```python
from build123d import *

# Parameters (mm, degrees)
SKETCH_1_R               = 9.5
EXTRUDE_2_DEPTH          = 10
CHAMFER_1_SIZE           = 0.5
CUT_EXTRUDE_1_DEPTH      = 10
SKETCH_3_R               = 2
CUT_EXTRUDE_2_DEPTH      = 10
CHAMFER_2_SIZE           = 0.5
SKETCH_5_R               = 2
CUT_EXTRUDE_3_DEPTH      = 10
CHAMFER_3_SIZE           = 0.5
SKETCH_9_R               = 2
EXTRUDE_3_DEPTH          = 10
SKETCH_10_R              = 2
CUT_EXTRUDE_6_DEPTH      = 10
PATTERN_CIRCULAR_2_COUNT = 4
SKETCH_11_R              = 1.5
CUT_EXTRUDE_7_DEPTH      = 251.99800796


with BuildPart() as part:
    # Sketch 1 → Extrude 2 (new body)
    with BuildSketch(Plane.XY):
        with BuildLine():
            Line((20.821645942, -9.5), (202.986114682, -9.5))
            ThreePointArc((202.986114682, -9.5), (210.231803055, -10.858648118), (216.493057341, -14.75))
            ThreePointArc((216.493057341, -14.75), (250, 0), (216.493057341, 14.75))
            ThreePointArc((216.493057341, 14.75), (210.231803055, 10.858648118), (202.986114682, 9.5))
            Line((202.986114682, 9.5), (21.63860854, 9.5))
            Line((21.63860854, 9.5), (16.904141504, 9.5))
            ThreePointArc((16.904141504, 9.5), (11.75918395, 10.173090993), (6.960528855, 12.147058824))
            ThreePointArc((6.960528855, 12.147058824), (3.490452231, 13.557903349), (-0.229510749, 13.998118617))
            ThreePointArc((-0.229510749, 13.998118617), (-13.878745314, -1.838594167), (3.423256182, -13.575025492))
            ThreePointArc((3.423256182, -13.575025492), (5.240755683, -12.982083033), (6.960528855, -12.147058824))
            ThreePointArc((6.960528855, -12.147058824), (11.75918395, -10.173090993), (16.904141504, -9.5))
            Line((16.904141504, -9.5), (20.821645942, -9.5))
        make_face()
        Circle(SKETCH_1_R, mode=Mode.SUBTRACT)
        with Locations((230, 0)):
            Circle(SKETCH_1_R, mode=Mode.SUBTRACT)
    extrude(amount=EXTRUDE_2_DEPTH)

    # Chamfer 1
    chamfer_1_edges = [part.edges().sort_by_distance(p)[0] for p in [
        (-9.5, 0, 0),
        (-9.5, 0, 10),
    ]]
    chamfer(chamfer_1_edges, length=CHAMFER_1_SIZE)

    # Sketch 2 → Cut-Extrude 1 (cut)
    with BuildSketch(Plane.XY.offset(10)):
        with BuildLine():
            Line((92.5, -6), (137.5, -6))
            ThreePointArc((137.5, -6), (143.5, 0), (137.5, 6))
            Line((137.5, 6), (92.5, 6))
            ThreePointArc((92.5, 6), (86.5, 0), (92.5, -6))
        make_face()
        with BuildLine():
            Line((157.5, -6), (202.5, -6))
            ThreePointArc((202.5, -6), (208.5, 0), (202.5, 6))
            Line((202.5, 6), (157.5, 6))
            ThreePointArc((157.5, 6), (151.5, 0), (157.5, -6))
        make_face()
        with BuildLine():
            Line((35, -6), (72.5, -6))
            ThreePointArc((72.5, -6), (78.5, 0), (72.5, 6))
            Line((72.5, 6), (35, 6))
            ThreePointArc((35, 6), (29, 0), (35, -6))
        make_face()
    extrude(amount=-CUT_EXTRUDE_1_DEPTH, mode=Mode.SUBTRACT)

    # Sketch 3 → Cut-Extrude 2 (cut)
    with BuildSketch(Plane.XY.offset(10)):
        with Locations((245, 0)):
            Circle(SKETCH_3_R)
        with Locations((237.5, 12.990381057)):
            Circle(SKETCH_3_R)
        with Locations((222.5, 12.990381057)):
            Circle(SKETCH_3_R)
    extrude(amount=-CUT_EXTRUDE_2_DEPTH, mode=Mode.SUBTRACT)

    # Chamfer 2
    chamfer_2_edges = [part.edges().sort_by_distance(p)[0] for p in [
        (220.5, 0, 10),
    ]]
    chamfer(chamfer_2_edges, length=CHAMFER_2_SIZE)

    # Sketch 5 → Cut-Extrude 3 (cut)
    with BuildSketch(Plane.XY.offset(10)):
        with Locations((215, 0)):
            Circle(SKETCH_5_R)
        with Locations((222.5, -12.990381057)):
            Circle(SKETCH_5_R)
        with Locations((237.5, -12.990381057)):
            Circle(SKETCH_5_R)
    extrude(amount=-CUT_EXTRUDE_3_DEPTH, mode=Mode.SUBTRACT)

    # Chamfer 3
    chamfer_3_edges = [part.edges().sort_by_distance(p)[0] for p in [
        (220.5, 0, 0),
    ]]
    chamfer(chamfer_3_edges, length=CHAMFER_3_SIZE)

    # Sketch 9 → Extrude 3 (add)
    with BuildSketch(Plane.XY.offset(10)):
        with Locations((215, 0)):
            Circle(SKETCH_9_R)
        with Locations((222.5, 12.990381057)):
            Circle(SKETCH_9_R)
        with Locations((237.5, 12.990381057)):
            Circle(SKETCH_9_R)
        with Locations((245, 0)):
            Circle(SKETCH_9_R)
        with Locations((237.5, -12.990381057)):
            Circle(SKETCH_9_R)
        with Locations((222.5, -12.990381057)):
            Circle(SKETCH_9_R)
    extrude(amount=-EXTRUDE_3_DEPTH)

    # Sketch 10 → Cut-Extrude 6 (cut)
    with BuildSketch(Plane.XY.offset(10)):
        with Locations((214.5, 0)):
            Circle(SKETCH_10_R)
    cut_extrude_6 = extrude(amount=-CUT_EXTRUDE_6_DEPTH, mode=Mode.SUBTRACT)

    # Pattern Circular 2: Cut-Extrude 6 ×4 about axis
    pattern_circular_2_axis = Axis((230, 0, 0), (0, 0, 1))
    for i in range(1, PATTERN_CIRCULAR_2_COUNT):
        add(cut_extrude_6.rotate(pattern_circular_2_axis, i * 360 / PATTERN_CIRCULAR_2_COUNT), mode=Mode.SUBTRACT)

    # Sketch 11 → Cut-Extrude 7 (cut, through all)
    with BuildSketch(Plane.XY.offset(10)):
        with Locations((17, 4)):
            Circle(SKETCH_11_R)
        with Locations((17, -4)):
            Circle(SKETCH_11_R)
    extrude(amount=-CUT_EXTRUDE_7_DEPTH, mode=Mode.SUBTRACT)


solid = part.part
```
CAD build for the part. Positions are in the model's coordinates, mm. A direction names the side the tool comes from. Give positions to 0.01 mm unless a question says otherwise; leave off trailing zeros. Write each loop counter-clockwise with the first axis right and the second up, starting at its lowest first coordinate (ties: lowest second). Pieces come first, ordered by that corner, then holes. Notation, with made-up numbers: M 1.5,43 L 26.5,43 A21 ccw 26.5,57 Z; hole C 22.5,-28.5 d7. An arc over 180 degrees is marked long. Return JSON: item names as keys, results as strings. Group by question number.
(1) Drill centre lines: L1, parallel to Y at x = 230, z = 3; L2, parallel to Y at x = 17, z = 4.5; L3, parallel to Y at x = 47.5, z = 9. Where is each one in solid material? Low to high. Write a range as [from, to].
(2) Band-saw the part on C-C (x = 148). Give the cut face in (y, z), and give its area (3 significant figures).
(3) 3-axis set-ups, long thin cutter, end or side, ignore diameter. For faces 1 (the face through (180, -6, 5)), 2 (the face through (109, -9.5, 5)), 3 (the face through (127, -7, 10)): which of +Z, -Z, +X, -X, +Y, -Y reach the whole face in a straight line?
(4) Band-saw the part on B-B (x = 102.5). Give the cut face in (y, z), and give its area (3 significant figures).
(5) Band-saw the part on A-A (z = 5.75). State how many separate pieces and enclosed holes the cut face has, and give its area (3 significant figures).
(6) Flat gauge pins, fed straight in: pin 1 Ø4.5 at (x, y) = (245.5, 0) entering from -Z; pin 2 Ø3 at (x, z) = (61.5, 6.5) entering from +Y; pin 3 Ø3 at (x, z) = (101.5, 4.5) entering from -Y; pin 4 Ø1.5 at (y, z) = (11.5, 8.5) entering from +X. Where does each tip first touch, or does it go through?
(7) Mould opens along Y. For faces 4 (the face through (127, -7, 0)), 5 (the face through (111, 9.5, 5)), 6 (the face through (78.5, -0.1, 5.1)), 7 (the face through (53, -6, 5)) say: pulls with the +Y half, pulls with the -Y half, needs draft (parallel to the pull), parting line crosses it, or undercut.
Entries:
{
 "1": {"L1": "y = [-20, -17.5], [-13.5, -9.5], [9.5, 13.5], [17.5, 20]", "L2": "y = [-9.5, -5.5], [-2.5, 2.5], [5.5, 9.5]", "L3": "y = [-9.5, -6], [6, 9.5]"},
 "2": {"outline": "M -9.5,0 L 9.5,0 L 9.5,10 L -9.5,10 Z", "area": "190 mm^2"},
 "3": {"face 1": "+Z, -Z", "face 2": "+Z, -Z, -Y", "face 3": "+Z, +X, -X, +Y, -Y"},
 "4": {"outline": "M -9.5,0 L -6,0 L -6,10 L -9.5,10 Z; M 6,0 L 9.5,0 L 9.5,10 L 6,10 Z", "area": "70.0 mm^2"},
 "5": {"separate pieces": "1", "enclosed holes": "11", "area": "3,160 mm^2"},
 "6": {"pin 1": "stops at z = 0", "pin 2": "stops at y = 9.5", "pin 3": "stops at y = -9.5", "pin 4": "stops at x = 246.87"},
 "7": {"face 4": "needs draft", "face 5": "pulls with the +Y half", "face 6": "undercut", "face 7": "undercut"}
}
